```python
from build123d import *

# Parameters (mm, degrees)
SKETCH_1_R      = 0.55
EXTRUDE_1_DEPTH = 3


with BuildPart() as part:
    # Эскиз1 → Бобышка-Вытянуть1 (new body)
    with BuildSketch(Plane(origin=(0, 0, 0), x_dir=(0, 0, -1), z_dir=(1, 0, 0))):
        with BuildLine():
            Line((4, 0), (6, 0))
            ThreePointArc((6, 0), (8.828427125, 1.171572875), (10, 4))
            Line((10, 4), (10, 36))
            ThreePointArc((10, 36), (8.828427125, 38.828427125), (6, 40))
            Line((6, 40), (4, 40))
            ThreePointArc((4, 40), (1.171572875, 38.828427125), (0, 36))
            Line((0, 36), (0, 4))
            ThreePointArc((0, 4), (1.171572875, 1.171572875), (4, 0))
        make_face()
        with Locations((5, 3)):
            Circle(SKETCH_1_R, mode=Mode.SUBTRACT)
        with Locations((5, 37)):
            Circle(SKETCH_1_R, mode=Mode.SUBTRACT)
        with BuildLine():
            Line((1.95, 35.75), (1.95, 34.25))
            ThreePointArc((1.95, 34.25), (1.2, 33.5), (0.45, 34.25))
            Line((0.45, 34.25), (0.45, 35.75))
            ThreePointArc((0.45, 35.75), (1.2, 36.5), (1.95, 35.75))
        make_face(mode=Mode.SUBTRACT)
        with BuildLine():
            Line((0.45, 4.25), (0.45, 5.75))
            ThreePointArc((0.45, 5.75), (1.2, 6.5), (1.95, 5.75))
            Line((1.95, 5.75), (1.95, 4.25))
            ThreePointArc((1.95, 4.25), (1.2, 3.5), (0.45, 4.25))
        make_face(mode=Mode.SUBTRACT)
        with BuildLine():
            Line((8.05, 4.25), (8.05, 5.75))
            ThreePointArc((8.05, 5.75), (8.8, 6.5), (9.55, 5.75))
            Line((9.55, 5.75), (9.55, 4.25))
            ThreePointArc((9.55, 4.25), (8.8, 3.5), (8.05, 4.25))
        make_face(mode=Mode.SUBTRACT)
        with BuildLine():
            Line((8.05, 34.25), (8.05, 35.75))
            ThreePointArc((8.05, 35.75), (8.8, 36.5), (9.55, 35.75))
            Line((9.55, 35.75), (9.55, 34.25))
            ThreePointArc((9.55, 34.25), (8.8, 33.5), (8.05, 34.25))
        make_face(mode=Mode.SUBTRACT)
    extrude(amount=EXTRUDE_1_DEPTH)


solid = part.part
```
Geometry: final body of the model. Coordinates: model frame, mm. A direction names the side the tool comes from. Round coordinates to 2 decimals unless told otherwise and drop trailing zeros. Loops run counter-clockwise (first coordinate to the right, second up) from the corner with the lowest first, then second, coordinate; pieces in that order, holes last. Notation, with made-up numbers: (-17.75, 32.5) -> (36.25, 32.5) arc R23 ccw to (36.25, 58.5) -> close; hole circle Ø9 at (44.5, -32). An arc over 180 degrees is marked (long way). Use one line per item in the form item = value. Start each with the question number.
1) Line query: L1, parallel to Z at x = 0.45, y = 5.5; L2, parallel to Y at x = 1.15, z = -5; L3, parallel to Y at x = 2.6, z = -1.5. Output: solid intervals per line, ascending.
2) First-contact query: P1, Ø1.4, axis at y = 37, z = -5, coming from the -X side; P2, Ø1.5, axis at x = 1.5, z = -9, coming from the +Y side. Flat tips, straight axial feed; report the tip coordinate or a pass-through.
3) Section C-C on z = -5. Output: boundary loops of the cut face in (x, y), then the cut area to 3 significant figures.
4) Access query for faces 4 (the flat face through (3, 20, -5)), 5 (the cylindrical face through (1.5, 33.5, -8.8)). Directions: +Z, -Z, +X, -X, +Y, -Y. A direction counts if a zero-diameter tool reaches every point of the face in a straight line with its end or side. Return the directions, or none.
5) Draft query along Y for faces 1 (the flat face through (1, 0, -5)), 2 (the cylindrical face through (1.479, 38.797, -8.859)), 3 (the flat face through (1, 35, -0.45)). Return one class per face: released by +Y, released by -Y, zero draft, split by the parting line, or undercut.
6) Section B-B on y = 3. Output: boundary loops of the cut face in (x, z).
7) Section D-D on z = -8.8. Output: boundary loops of the cut face in (x, y), then the cut area to 3 significant figures.
8) Section A-A on x = 0.75. Output: boundary loops of the cut face in (y, z).
Response:
q1.L1 = -10 to -9.55, -8.05 to -1.95, -0.45 to 0
q1.L2 = 0 to 2.45, 3.55 to 36.45, 37.55 to 40
q1.L3 = 0.88 to 3.56, 6.44 to 33.56, 36.44 to 39.12
q2.P1 = 0
q2.P2 = 39.31
q3.outline = (0, 0) -> (3, 0) -> (3, 2.45) -> (0, 2.45) -> close; (0, 3.55) -> (3, 3.55) -> (3, 36.45) -> (0, 36.45) -> close; (0, 37.55) -> (3, 37.55) -> (3, 40) -> (0, 40) -> close
q3.area = 113 mm^2
q4.face_4 = +Z, -Z, +X, +Y, -Y
q4.face_5 = +X, -X
q5.face_1 = released by -Y
q5.face_2 = released by +Y
q5.face_3 = undercut
q6.outline = (0, -9.87) -> (3, -9.87) -> (3, -5.55) -> (0, -5.55) -> close; (0, -4.45) -> (3, -4.45) -> (3, -0.13) -> (0, -0.13) -> close
q7.outline = (0, 1.14) -> (3, 1.14) -> (3, 3.5) -> (0, 3.5) -> close; (0, 6.5) -> (3, 6.5) -> (3, 33.5) -> (0, 33.5) -> close; (0, 36.5) -> (3, 36.5) -> (3, 38.86) -> (0, 38.86) -> close
q7.area = 95.1 mm^2
q8.outline = (0, -6) arc R4 ccw to (4, -10) -> (36, -10) arc R4 ccw to (40, -6) -> (40, -4) arc R4 ccw to (36, 0) -> (4, 0) arc R4 ccw to (0, -4) -> close; hole circle Ø1.1 at (3, -5); hole (4.25, -9.55) -> (5.75, -9.55) arc R0.75 ccw to (5.75, -8.05) -> (4.25, -8.05) arc R0.75 ccw to start; hole (4.25, -1.95) -> (5.75, -1.95) arc R0.75 ccw to (5.75, -0.45) -> (4.25, -0.45) arc R0.75 ccw to start; hole (34.25, -9.55) -> (35.75, -9.55) arc R0.75 ccw to (35.75, -8.05) -> (34.25, -8.05) arc R0.75 ccw to start; hole (34.25, -1.95) -> (35.75, -1.95) arc R0.75 ccw to (35.75, -0.45) -> (34.25, -0.45) arc R0.75 ccw to start; hole circle Ø1.1 at (37, -5)
